Can you work these out from the model? Positions are in its coordinate system, mm. Give positions to 0.01 mm unless a question says otherwise; leave off trailing zeros. Order: outer loops, then holes, each group sorted by start corner. A loop starts at its lowest first (then second) coordinate and runs counter-clockwise, first axis right, second up. Notation, with made-up numbers: (80, -10) - (115, -10) arc R20 cw to (115, 19) - close; hole circle Ø1 at (78.5, 23.25). An arc over 180 degrees is marked (long way). Answer as CSV lines item,"result".
```python
from build123d import *

# Parameters (mm, degrees)
F2_SIZE2 = 2.54
F2_SIZE  = 0.635
F3_SIZE  = 0.635


with BuildPart() as f1:
    # F0 (on Front) → F1 (revolve)
    with BuildSketch(Plane.XZ):
        Polygon((-1.3462, 0), (0, 0), (0, 35.56), (-1.3462, 35.56), (-1.3462, 12.7), align=None)
    revolve(axis=Axis((0, 0, 17.78), (0, 0, 1)))

    # F2
    f2_edges = [f1.edges().sort_by_distance(p)[0] for p in [
        (1.3462, 0, 0),
    ]]
    chamfer(f2_edges, length=F2_SIZE, length2=F2_SIZE2)

    # F3
    f3_edges = [f1.edges().sort_by_distance(p)[0] for p in [
        (1.3462, 0, 35.56),
    ]]
    chamfer(f3_edges, length=F3_SIZE)


solid = f1.part
```
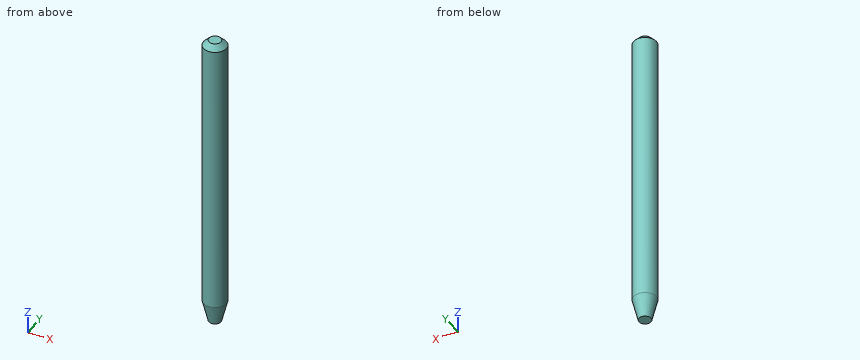
1) I want a section at A-A on x = 0. Write out the boundary of the cut face in (y, z) (3 decimals), plus the area to 3 significant figures.
Answer block:
outline,"(-1.346, 2.54) - (-0.711, 0) - (0.711, 0) - (1.346, 2.54) - (1.346, 34.925) - (0.711, 35.56) - (-0.711, 35.56) - (-1.346, 34.925) - close"
area,"93.7 mm2"
2) I need wall thicknesses on line 1 along X through (y, z) = (0.7, 9); line 2 along X through (y, z) = (-0.4, 29.5); line 3 along Y through (x, z) = (-1.1, 10). Which ranges of each line are inside material? Lowest first, please. Write a range as [from, to].
Answer block:
line 1,"[-1.15, 1.15]"
line 2,"[-1.29, 1.29]"
line 3,"[-0.78, 0.78]"
3) I want a section at C-C on z = 19.5. Write out the boundary of the cut face in (x, y).
Answer block:
outline,"circle Ø2.69 at (0, 0)"
